```python
from build123d import *

# Parameters (mm, degrees)
SKETCH1_R           = 8
BOSS_EXTRUDE1_DEPTH = 27.5
SKETCH2_W           = 49
SKETCH2_H           = 60
BOSS_EXTRUDE2_DEPTH = 45
SKETCH3_R           = 16
BOSS_EXTRUDE3_DEPTH = 30
SKETCH4_W           = 49
SKETCH4_H           = 45
BOSS_EXTRUDE4_DEPTH = 47.5
BOSS_EXTRUDE5_DEPTH = 49
SKETCH6_W           = 24.794244746
SKETCH6_H           = 50
CUT_EXTRUDE1_DEPTH  = 81
SKETCH7_R           = 6
CUT_EXTRUDE2_DEPTH  = 53
SKETCH8_R           = 6
BOSS_EXTRUDE6_DEPTH = 49
FILLET1_R           = 5
FILLET2_R           = 5
FILLET4_R           = 3
CUT_EXTRUDE4_DEPTH  = 81
SKETCH12_R          = 6
BOSS_EXTRUDE7_DEPTH = 32


with BuildPart() as part:
    # Sketch1 → Boss-Extrude1 (new body, symmetric)
    with BuildSketch(Plane(origin=(0, 0, 0), x_dir=(0, 0, -1), z_dir=(1, 0, 0))):
        with BuildLine():
            Line((-17.5, 0), (-17.5, 17.5))
            Line((-17.5, 17.5), (17.5, 17.5))
            Line((17.5, 17.5), (17.5, 0))
            ThreePointArc((17.5, 0), (0, -17.5), (-17.5, 0))
        make_face()
        Circle(SKETCH1_R, mode=Mode.SUBTRACT)
    extrude(amount=BOSS_EXTRUDE1_DEPTH, both=True)

    # Sketch2 → Boss-Extrude2 (add)
    with BuildSketch(Plane(origin=(0, 17.5, 0), x_dir=(1, 0, 0), z_dir=(0, 1, 0))):
        with Locations((0, 14.5)):
            Rectangle(SKETCH2_W, SKETCH2_H)
    extrude(amount=BOSS_EXTRUDE2_DEPTH)

    # Sketch3 → Boss-Extrude3 (add)
    with BuildSketch(Plane(origin=(0, 0, -44.5), x_dir=(-1, 0, 0), z_dir=(0, 0, -1))):
        with Locations((0, 40)):
            Circle(SKETCH3_R)
    extrude(amount=BOSS_EXTRUDE3_DEPTH)

    # Sketch4 → Boss-Extrude4 (add)
    with BuildSketch(Plane(origin=(0, 0, -74.5), x_dir=(-1, 0, 0), z_dir=(0, 0, -1))):
        with Locations((0, 40)):
            Rectangle(SKETCH4_W, SKETCH4_H)
    extrude(amount=BOSS_EXTRUDE4_DEPTH)

    # Sketch5 → Boss-Extrude5 (add)
    with BuildSketch(Plane(origin=(24.5, 0, 0), x_dir=(0, 0, -1), z_dir=(1, 0, 0))):
        with BuildLine():
            Line((122, 62.5), (122, 17.5))
            ThreePointArc((122, 17.5), (144.5, 40), (122, 62.5))
        make_face()
    extrude(amount=-BOSS_EXTRUDE5_DEPTH)

    # Sketch6 → Cut-Extrude1 (cut, through all)
    with BuildSketch(Plane(origin=(0, 62.5, 0), x_dir=(1, 0, 0), z_dir=(0, 1, 0))):
        with Locations((0, 119.5)):
            Rectangle(SKETCH6_W, SKETCH6_H)
    extrude(amount=-CUT_EXTRUDE1_DEPTH, mode=Mode.SUBTRACT)

    # Sketch7 → Cut-Extrude2 (cut, through all)
    with BuildSketch(Plane(origin=(24.5, 0, 0), x_dir=(0, 0, -1), z_dir=(1, 0, 0))):
        with Locations((122, 40)):
            Circle(SKETCH7_R)
    extrude(amount=-CUT_EXTRUDE2_DEPTH, mode=Mode.SUBTRACT)

    # Sketch8 → Boss-Extrude6 (add)
    with BuildSketch(Plane(origin=(24.5, 0, 0), x_dir=(0, 0, -1), z_dir=(1, 0, 0))):
        with Locations((122, 40)):
            Circle(SKETCH8_R)
    extrude(amount=-BOSS_EXTRUDE6_DEPTH)

    # Fillet1
    fillet1_edges = [part.edges().sort_by_distance(p)[0] for p in [
        (16, 40, -44.5),
    ]]
    fillet(fillet1_edges, radius=FILLET1_R)

    # Fillet2
    fillet2_edges = [part.edges().sort_by_distance(p)[0] for p in [
        (16, 40, -74.5),
    ]]
    fillet(fillet2_edges, radius=FILLET2_R)

    # Fillet4
    fillet4_edges = [part.edges().sort_by_distance(p)[0] for p in [
        (0, 62.5, 15.5),
    ]]
    fillet(fillet4_edges, radius=FILLET4_R)

    # Sketch10 → Cut-Extrude4 (cut, through all)
    with BuildSketch(Plane(origin=(0, 62.5, 0), x_dir=(1, 0, 0), z_dir=(0, 1, 0))):
        Polygon((16, 94.5), (16, 144.5), (-16, 144.5), (-16, 97.685176626), (-16, 94.5), align=None)
    extrude(amount=-CUT_EXTRUDE4_DEPTH, mode=Mode.SUBTRACT)

    # Sketch12 → Boss-Extrude7 (add)
    with BuildSketch(Plane.ZY.offset(-16)):
        with Locations((-122, 40)):
            Circle(SKETCH12_R)
    extrude(amount=BOSS_EXTRUDE7_DEPTH)


solid = part.part
```
Work out the finished part from the listing and answer in its coordinate system (mm). A direction names the side the tool comes from. Give positions to 0.01 mm unless a question says otherwise; leave off trailing zeros. Loops run counter-clockwise (first coordinate to the right, second up) from the corner with the lowest first, then second, coordinate; pieces in that order, holes last. Notation, with made-up numbers: M -35,38 L -30,38 A30 cw -30,69 Z; hole C 34.5,-29 d9. An arc over 180 degrees is marked long. One line per item, written item: value. Start each with the question number.
1. Find section D-D (y = -3.5). Give the vertices of the cut face in (x, z).
2. Determine the mould class of faces 5 (the face through (0, 9, -17.5)), 6 (the face through (0, 62.5, -16)), 7 (the face through (-0.39, -7.81, 1.73)), 8 (the face through (0.385, -17.496, -0.385)) for opening direction Y: released by +Y, released by -Y, zero draft, split by the parting line, or undercut.
3. Which of the six approach directions +Z, -Z, +X, -X, +Y, -Y give full straight-line access (tool end or side, diameter ignored) to faces 1 (the face through (0, 40, -94.5)), 2 (the face through (-22, 40, -44.5)), 3 (the face through (0, 17.5, -93)), 4 (the face through (0, 38, 15.5))?
4. Each of these flat-tipped pins is pushed along its axis until it touches: P1, Ø22.5, axis at y = 40, z = -28.5, coming from the -X side; P2, Ø14, axis at x = -7.5, y = 9, coming from the -Z side; P3, Ø4, axis at x = 21, y = 23, coming from the +Z side. Where does it stop, or does it pass through?
5. Find the intervals of material crossed by probe 1 along Y at (x, z) = (-9, 0); probe 2 along X at (y, z) = (52, -102); probe 3 along X at (y, z) = (59, -84), in increasing order.
6. Find section B-B (z = 0). Give the vertices of the cut face in (x, y).
7. Find section C-C (y = 40). Give the vertices of the cut face in (x, z).
8. Find section A-A (x = 0). Give the vertices of the cut face in (y, z).
Reported:
1. outline: M -27.5,-17.15 L 27.5,-17.15 L 27.5,-7.19 L -27.5,-7.19 Z; M -27.5,7.19 L 27.5,7.19 L 27.5,17.15 L -27.5,17.15 Z
2. face 5: zero draft
2. face 6: released by +Y
2. face 7: undercut
2. face 8: released by -Y
3. face 1: +Y, -Y
3. face 2: none
3. face 3: -Z, +X, -X, -Y
3. face 4: +Z, +X, -X, +Y
4. P1: stops at x = -24.5
4. P2: stops at z = -17.5
4. P3: stops at z = 15.5
5. probe 1: y = -17.5 to -8, 8 to 62.5
5. probe 2: x = -24.5 to -16, 16 to 24.5
5. probe 3: x = -24.5 to 24.5
6. outline: M -27.5,-17.5 L 27.5,-17.5 L 27.5,-8 L -27.5,-8 Z; M -27.5,8 L 27.5,8 L 27.5,17.5 L 24.5,17.5 L 24.5,62.5 L -24.5,62.5 L -24.5,17.5 L -27.5,17.5 Z
7. outline: M -24.5,-144.5 L -16,-144.5 L -16,-128 L 16,-128 L 16,-144.5 L 24.5,-144.5 L 24.5,-74.5 L 21,-74.5 A5 cw 16,-69.5 L 16,-49.5 A5 cw 21,-44.5 L 24.5,-44.5 L 24.5,15.5 L -24.5,15.5 L -24.5,-44.5 L -21,-44.5 A5 cw -16,-49.5 L -16,-69.5 A5 cw -21,-74.5 L -24.5,-74.5 Z; hole M -16,-116 L 16,-116 L 16,-94.5 L -16,-94.5 Z
8. outline: M 0,-17.5 L 17.5,-17.5 L 17.5,-44.5 L 19,-44.5 A5 cw 24,-49.5 L 24,-69.5 A5 cw 19,-74.5 L 17.5,-74.5 L 17.5,-94.5 L 62.5,-94.5 L 62.5,-74.5 L 61,-74.5 A5 cw 56,-69.5 L 56,-49.5 A5 cw 61,-44.5 L 62.5,-44.5 L 62.5,12.5 A3 ccw 59.5,15.5 L 17.5,15.5 L 17.5,17.5 L 0,17.5 A17.5 ccw Z; C 40,-122 d12; hole C 0,0 d16
